Source: CAD feature listing. Evaluate the final solid. Frame: model axes, mm. Face numbers are marked on the shaded views. A direction names the side the tool comes from. Give positions to 0.01 mm unless a question says otherwise; leave off trailing zeros. Loops run counter-clockwise (first coordinate to the right, second up) from the corner with the lowest first, then second, coordinate; pieces in that order, holes last. Notation, with made-up numbers: M -19.5,-0.75 L 16.5,-0.75 A21 ccw 16.5,13.25 Z; hole C 14,41 d11. An arc over 180 degrees is marked long. Answer in a Markdown table with one row per item.
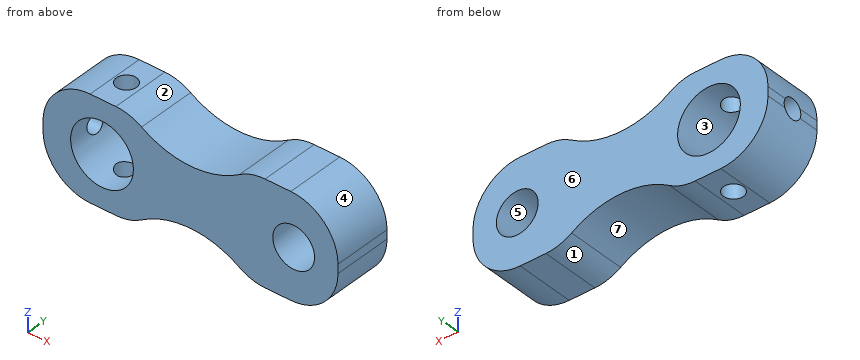
Autodesk Inventor part; units mm, degrees
ref_plane "YZ Plane" through (0, 0, 0) normal (1, 0, 0) x (0, 1, 0)
ref_plane "XZ Plane" through (0, 0, 0) normal (0, 1, 0) x (-1, 0, 0)
ref_plane "XY Plane" through (0, 0, 0) normal (0, 0, 1) x (1, 0, 0)
sketch "Sketch1" plane through (0, 0, 0) normal (0, 1, 0) x (-1, 0, 0)
  line L0 (15.875, 5.5563) -> (-15.875, 5.5563)
  line L1 (-15.875, 5.5563) -> (-15.875, -5.5563)
  line L2 (-15.875, -5.5563) -> (15.875, -5.5563)
  line L3 (15.875, -5.5563) -> (15.875, 5.5563)
  point P0 (0, 0)
  dimension "d0" = 31.75
  dimension "d1" = 11.1125
extrude "Extrusion1" add sketch "Sketch1" along normal blind 6.35
sketch "Sketch2" plane through (0, 6.35, 0) normal (0, 1, 0) x (1, 0, 0)
  line L0 (15.875, -5.5563) -> (15.875, 5.5563)
  line L1 (15.875, 5.5563) -> (-15.875, 5.5563)
  point P0 (0, 0)
  point P1 (11.1125, 0)
  dimension "d4" = 4.7625
  dimension "d5" = 5.5563
hole "Hole1" at (11.1125, 6.35, 0) direction (0, -1, 0) diameter 4.4958 end through all
sketch "Sketch3" plane through (0, 6.35, 0) normal (0, 1, 0) x (1, 0, 0)
  line L0 (-15.875, 5.5563) -> (-15.875, -5.5563)
  line L1 (15.875, 5.5563) -> (-15.875, 5.5563)
  point P0 (0, 0)
  point P1 (-9.525, 0)
  dimension "d13" = 6.35
  dimension "d14" = 5.5563
hole "Hole2" at (-9.525, 6.35, 0) direction (0, -1, 0) diameter 6.7564 end through all
fillet "Fillet1" radius 5.08 4 edges at (15.875, 3.175, -5.5563) (15.875, 3.175, 5.5563) (-15.875, 3.175, -5.5563) (-15.875, 3.175, 5.5563)
sketch "Sketch4" plane through (0, 6.35, 0) normal (0, 1, 0) x (1, 0, 0)
  line L0 (-10.795, -5.5563) -> (10.795, -5.5563)
  arc A0 (6.35, -5.5563) -> (-6.35, -5.5563) centre (0, -12.8323) ccw
  line L1 (10.795, 5.5563) -> (-10.795, 5.5563)
  arc A1 (-6.35, 5.5563) -> (6.35, 5.5563) centre (0, 12.8323) ccw
  point P0 (0, 0)
  dimension "d23" = 12.7
  dimension "d24" = 12.7
extrude "Extrusion2" cut sketch "Sketch4" against normal blind 6.35
fillet "Fillet2" radius 5.08 4 edges at (-6.35, 3.175, -5.5563) (6.35, 3.175, -5.5563) (-6.35, 3.175, 5.5563) (6.35, 3.175, 5.5563)
sketch "Sketch5" plane through (-10.795, 0, 5.5563) normal (0, 0, 1) x (1, 0, 0)
  line L0 (0, 6.35) -> (2.7628, 6.35)
  line L1 (-5.08, 6.35) -> (-5.08, 0)
  point P0 (10.795, 0)
  point P1 (1.27, 3.175)
  dimension "d28" = 3.175
  dimension "d29" = 6.35
hole "Hole3" at (-9.525, 3.175, 5.5563) direction (0, 0, -1) diameter 2.1565 end through all
sketch "Sketch6" plane through (-15.875, 0, -0.4763) normal (-1, 0, 0) x (0, 0, 1)
  line L0 (0, 6.35) -> (0.9525, 6.35)
  line L1 (-5.08, 6.35) -> (-5.08, 0)
  point P0 (0.4763, 0)
  point P1 (0.4474, 3.175)
  dimension "d37" = 3.175
  dimension "d38" = 5.5274
hole "Hole4" at (-15.875, 3.175, -0.0288) direction (1, 0, 0) diameter 2.1565 end up to surface
properties part number "Tube to TRB1 adapter"
Q1. Reachability of the marked faces 1, 2 and 3 from +Z, -Z, +X, -X, +Y, -Y: full face, straight path, thin tool, end or side. Return the list, or none.
Values follow:
| item | result |
|---|---|
| face 1 | -Z, +Y, -Y |
| face 2 | +Z, +Y, -Y |
| face 3 | +Y, -Y |
Q2. Mould query, pull axis Z, two halves, no side actions, for the marked faces 4, 5, 6 and 7. Classes: +Z half, -Z half, draft (parallel to the pull), parting line (faces both ways), or undercut.
Values follow:
| item | result |
|---|---|
| face 4 | +Z half |
| face 5 | undercut |
| face 6 | draft |
| face 7 | -Z half |
Q3. Contact query for flat-ended pins moving along their axis: pin 1 Ø4 at (x, z) = (-9.525, 0) entering from +Y; pin 2 Ø1 at (y, z) = (4, 2) entering from -X. Output: stop coordinate, or through.
Values follow:
| item | result |
|---|---|
| pin 1 | through |
| pin 2 | x = -15.77 |
Q4. Section query A-A (x = -10). Output: boundary loops of the cut face in (y, z), plus the area to 3 significant figures.
Values follow:
| item | result |
|---|---|
| outline | M 0,-5.56 L 2.21,-5.56 L 2.21,-3.34 L 0,-3.34 Z; M 0,3.34 L 2.21,3.34 L 2.21,5.56 L 0,5.56 Z; M 4.14,-5.56 L 6.35,-5.56 L 6.35,-3.34 L 4.14,-3.34 Z; M 4.14,3.34 L 6.35,3.34 L 6.35,5.56 L 4.14,5.56 Z |
| area | 19.5 mm^2 |
Q5. Ray query, probe 1 along X at (y, z) = (4.5, 0) (3 decimals); probe 2 along X at (y, z) = (3.25, 0) (3 decimals); probe 3 along X at (y, z) = (4.75, -1.5). Return the intervals inside material, ascending. Write a range as from..to.
Values follow:
| item | result |
|---|---|
| probe 1 | -15.875..-12.903, -6.147..8.865, 13.36..15.875 |
| probe 2 | -6.147..8.865, 13.36..15.875 |
| probe 3 | -15.77..-12.55, -6.5..9.44, 12.79..15.77 |
Q6. Section query C-C (y = 5.25). Output: boundary loops of the cut face in (x, z) (1 decimal).
Values follow:
| item | result |
|---|---|
| outline | M -15.9,-0.5 A5.1 ccw -10.8,-5.6 L -8,-5.6 A5.1 ccw -5.3,-4.7 A9.7 cw 5.3,-4.7 A5.1 ccw 8,-5.6 L 10.8,-5.6 A5.1 ccw 15.9,-0.5 L 15.9,0.5 A5.1 ccw 10.8,5.6 L 8,5.6 A5.1 ccw 5.3,4.7 A9.7 cw -5.3,4.7 A5.1 ccw -8,5.6 L -10.8,5.6 A5.1 ccw -15.9,0.5 Z; hole C -9.5,0 d6.8; hole C 11.1,0 d4.5 |
Q7. Section query B-B (z = 0). Output: boundary loops of the cut face in (x, y) (3 decimals), plus the area to 3 significant figures.
Values follow:
| item | result |
|---|---|
| outline | M -15.875,0 L -12.903,0 L -12.903,2.097 L -15.875,2.097 Z; M -15.875,4.253 L -12.903,4.253 L -12.903,6.35 L -15.875,6.35 Z; M -6.147,0 L 8.865,0 L 8.865,6.35 L -6.147,6.35 Z; M 13.36,0 L 15.875,0 L 15.875,6.35 L 13.36,6.35 Z |
| area | 124 mm^2 |
